Here's how the part is built. I have some questions about the finished solid (model axes, mm). Round coordinates to 2 decimals unless told otherwise and drop trailing zeros. Loops run counter-clockwise (first coordinate to the right, second up) from the corner with the lowest first, then second, coordinate; pieces in that order, holes last. Notation, with made-up numbers: M 69.25,48 L 82.25,48 A8 cw 82.25,57 Z; hole C 81.25,-23 d11. An arc over 180 degrees is marked long. Use a Markdown table: item, result.
from build123d import *

# Parameters (mm, degrees)
SKETCH_1_W          = 54.8
SKETCH_1_H          = 54.8
SKETCH_1_R          = 6.5
SKETCH_1_R_2        = 1.6
SKETCH_1_W_2        = 4.4
SKETCH_1_H_2        = 8
SKETCH_1_W_3        = 8
SKETCH_1_H_3        = 4.4
EXTRUDE_1_DEPTH     = 4.4
FILLET_1_R          = 6
SKETCH_2_R          = 1.6
CUT_EXTRUDE_1_DEPTH = 10


with BuildPart() as part:
    # 草图1 → 凸台-拉伸1 (new body)
    with BuildSketch(Plane(origin=(0, 0, 0), x_dir=(1, 0, 0), z_dir=(0, 1, 0))):
        Rectangle(SKETCH_1_W, SKETCH_1_H)
        Circle(SKETCH_1_R, mode=Mode.SUBTRACT)
        with Locations((21.4, 21.4)):
            Circle(SKETCH_1_R_2, mode=Mode.SUBTRACT)
        with Locations((21.4, -21.4)):
            Circle(SKETCH_1_R_2, mode=Mode.SUBTRACT)
        with Locations((-21.4, -21.4)):
            Circle(SKETCH_1_R_2, mode=Mode.SUBTRACT)
        with Locations((-21.4, 21.4)):
            Circle(SKETCH_1_R_2, mode=Mode.SUBTRACT)
        with Locations((20.2, 9)):
            Rectangle(SKETCH_1_W_2, SKETCH_1_H_2, mode=Mode.SUBTRACT)
        with Locations((20.2, -9)):
            Rectangle(SKETCH_1_W_2, SKETCH_1_H_2, mode=Mode.SUBTRACT)
        with Locations((-20.2, -9)):
            Rectangle(SKETCH_1_W_2, SKETCH_1_H_2, mode=Mode.SUBTRACT)
        with Locations((-20.2, 9)):
            Rectangle(SKETCH_1_W_2, SKETCH_1_H_2, mode=Mode.SUBTRACT)
        with Locations((9, 20.2)):
            Rectangle(SKETCH_1_W_3, SKETCH_1_H_3, mode=Mode.SUBTRACT)
        with Locations((9, -20.2)):
            Rectangle(SKETCH_1_W_3, SKETCH_1_H_3, mode=Mode.SUBTRACT)
        with Locations((-9, -20.2)):
            Rectangle(SKETCH_1_W_3, SKETCH_1_H_3, mode=Mode.SUBTRACT)
        with Locations((-9, 20.2)):
            Rectangle(SKETCH_1_W_3, SKETCH_1_H_3, mode=Mode.SUBTRACT)
    extrude(amount=EXTRUDE_1_DEPTH)

    # 圆角1
    fillet_1_edges = [part.edges().sort_by_distance(p)[0] for p in [
        (27.4, 2.2, 27.4),
        (-27.4, 2.2, 27.4),
        (-27.4, 2.2, -27.4),
        (27.4, 2.2, -27.4),
    ]]
    fillet(fillet_1_edges, radius=FILLET_1_R)

    # 草图2 → 切除-拉伸1 (cut)
    with BuildSketch(Plane(origin=(0, 4.4, 0), x_dir=(1, 0, 0), z_dir=(0, 1, 0))):
        with Locations((10.7, 10.7)):
            Circle(SKETCH_2_R)
        with Locations((10.7, -10.7)):
            Circle(SKETCH_2_R)
        with Locations((-10.7, -10.7)):
            Circle(SKETCH_2_R)
        with Locations((-10.7, 10.7)):
            Circle(SKETCH_2_R)
    extrude(amount=-CUT_EXTRUDE_1_DEPTH, mode=Mode.SUBTRACT)


solid = part.part
1. Imagine slicing it at D-D, the plane y = 2.85. State how many separate pieces and enclosed holes the cut face has, then the cut area to 3 significant figures.
Answer sheet:
| item | result |
|---|---|
| separate pieces | 1 |
| enclosed holes | 17 |
| area | 2,490 mm2 |
2. Imagine slicing it at A-A, the plane x = 7.5. Write out the boundary of the cut face in (y, z), then the cut area to 3 significant figures.
Answer sheet:
| item | result |
|---|---|
| outline | M 0,-27.4 L 4.4,-27.4 L 4.4,-22.4 L 0,-22.4 Z; M 0,-18 L 4.4,-18 L 4.4,18 L 0,18 Z; M 0,22.4 L 4.4,22.4 L 4.4,27.4 L 0,27.4 Z |
| area | 202 mm2 |
3. I need wall thicknesses on probe 1 along Z at (x, y) = (10.7, 2.65); probe 2 along Z at (x, y) = (-19, 3.7); probe 3 along Z at (x, y) = (-21.4, 0.9). Which ranges of each line are inside material? Lowest first, please. Write a range as from..to.
Answer sheet:
| item | result |
|---|---|
| probe 1 | -27.4..-22.4, -18..-12.3, -9.1..9.1, 12.3..18, 22.4..27.4 |
| probe 2 | -27.4..-13, -5..5, 13..27.4 |
| probe 3 | -27.4..-23, -19.8..-13, -5..5, 13..19.8, 23..27.4 |
4. For pin 1 Ø2 at (x, z) = (15.5, -7) entering from -Y; pin 2 Ø10.5 at (x, z) = (0, 0) entering from -Y, each with a flat end and sliding along its axis, tell me the tip position at first contact or that it passes through.
Answer sheet:
| item | result |
|---|---|
| pin 1 | y = 0 |
| pin 2 | through |
5. We'd pull the mould along X, two halves only. Please class faces 1 (the face through (9, 2, -18)), 2 (the face through (25.596, 2.231, 25.689)): +X half, -X half, draft (parallel to the pull), parting line (faces both ways), or undercut.
Answer sheet:
| item | result |
|---|---|
| face 1 | undercut |
| face 2 | +X half |
6. Imagine slicing it at B-B, the plane z = -10.7. Write out the boundary of the cut face in (x, y), then the cut area to 3 significant figures.
Answer sheet:
| item | result |
|---|---|
| outline | M -27.4,0 L -22.4,0 L -22.4,4.4 L -27.4,4.4 Z; M -18,0 L -12.3,0 L -12.3,4.4 L -18,4.4 Z; M -9.1,0 L 9.1,0 L 9.1,4.4 L -9.1,4.4 Z; M 12.3,0 L 18,0 L 18,4.4 L 12.3,4.4 Z; M 22.4,0 L 27.4,0 L 27.4,4.4 L 22.4,4.4 Z |
| area | 174 mm2 |
7. Imagine slicing it at C-C, the plane x = 0. Write out the boundary of the cut face in (y, z), then the cut area to 3 significant figures.
Answer sheet:
| item | result |
|---|---|
| outline | M 0,-27.4 L 4.4,-27.4 L 4.4,-6.5 L 0,-6.5 Z; M 0,6.5 L 4.4,6.5 L 4.4,27.4 L 0,27.4 Z |
| area | 184 mm2 |
